```python
from build123d import *

# Parameters (mm, degrees)
F3_D     = 6.5278
F3_DEPTH = 9.525
F3_TIP   = 1.9611489744
F5_D     = 6.5278
F5_DEPTH = 9.525
F5_TIP   = 1.9611489744


with BuildPart() as f1:
    # F0 (on Front) → F1 (revolve)
    with BuildSketch(Plane.XZ):
        with BuildLine():
            Line((-57.0530471623, 106.8800194085), (-82.4530471623, 106.8800194085))
            Line((-82.4530471623, 106.8800194085), (-82.4530471623, -45.5199805915))
            Line((-82.4530471623, -45.5199805915), (-44.3530471623, -45.5199805915))
            Line((-44.3530471623, -45.5199805915), (-44.3530471623, -32.8199805915))
            add(Edge.make_bspline(
                [(-72.9280471623, -20.1199805915), (-72.9280471623, -32.8199805915), (-55.7276420295, -32.8199805915), (-44.3530471623, -32.8199805915)],
                knots=[0, 0, 0, 0, 31.2701235207, 31.2701235207, 31.2701235207, 31.2701235207], degree=3))
            Line((-72.9280471623, -20.1199805915), (-72.9280471623, 81.4800194085))
            ThreePointArc((-72.9280471623, 81.4800194085), (-69.2083032834, 90.4602755295), (-60.2280471623, 94.1800194085))
            Line((-60.2280471623, 94.1800194085), (-57.0530471623, 94.1800194085))
            Line((-57.0530471623, 94.1800194085), (-57.0530471623, 106.8800194085))
        make_face()
    revolve(axis=Axis((-82.4530471623, 0, 30.6800194085), (0, 0, -1)))

    # F3
    with Locations(Plane.XY.offset(106.8800194085)):
        with Locations((-82.4530471623, 15.875), (-82.4530471623, -15.875)):
            Hole(F3_D / 2, depth=F3_DEPTH)
            with Locations((0, 0, -(F3_DEPTH + F3_TIP / 2))):  # 118° drill point
                Cone(0, F3_D / 2, F3_TIP, mode=Mode.SUBTRACT)

    # F5
    with Locations(Plane(origin=(0, 0, -45.5199805915), x_dir=(1, 0, 0), z_dir=(0, 0, -1))):
        with Locations((-82.4530471623, 19.05), (-82.4530471623, -19.05)):
            Hole(F5_D / 2, depth=F5_DEPTH)
            with Locations((0, 0, -(F5_DEPTH + F5_TIP / 2))):  # 118° drill point
                Cone(0, F5_D / 2, F5_TIP, mode=Mode.SUBTRACT)


solid = f1.part
```
Here's how the part is built. I have some questions about the finished solid (model axes, mm). A direction names the side the tool comes from. Round coordinates to 2 decimals unless told otherwise and drop trailing zeros. Loops run counter-clockwise (first coordinate to the right, second up) from the corner with the lowest first, then second, coordinate; pieces in that order, holes last. Notation, with made-up numbers: (76, 18.25) -> (116, 18.25) arc R9 cw to (116, 22.25) -> close; hole circle Ø6 at (7, -4). An arc over 180 degrees is marked (long way). Answer as CSV lines item,"result". Start each with the question number.
1. I'm going to push flat-ended pins straight in: P1, Ø4, axis at x = -82.45, y = -19.05, coming from the +Z side; P2, Ø6, axis at y = -4, z = 68, coming from the -X side; P3, Ø10, axis at x = -101.5, z = 7, coming from the +Y side; P4, Ø5, axis at x = -82.45, y = 15.88, coming from the +Z side. Where does each tip first touch, or does it pass through?
2. Imagine slicing it at A-A on z = 52.5. Write out the boundary of the cut face in (x, y) (3 decimals), plus the area to 3 significant figures.
3. If we mould it in two halves opening along Z, with no side actions, what happens to faces 4 (the face through (-82.3, 22.5, 94.18)), 5 (the face through (-73.368, -2.861, 31.391)), 6 (the face through (-82.576, 19.603, -34.374)), 7 (the face through (-85.566, 16.855, 102.051))? For each: pulls with the +Z half, pulls with the -Z half, needs draft (parallel to the pull), parting line crosses it, or undercut.
4. I need wall thicknesses on probe 1 along Z at (x, y) = (-100, -16.5); probe 2 along X at (y, z) = (19, -43); probe 3 along Z at (x, y) = (-107.5, -22.5). Which ranges of each line are inside material? Lowest first, please. Write a range as from..to.
5. For faces 1 (the face through (-85.566, -20.03, -40.691)), 2 (the face through (-85.566, -14.895, 102.051)), 3 (the face through (-82, -1, -45.52)), which set-ups out of +Z, -Z, +X, -X, +Y, -Y let a thin tool reach every point of the face, with its end or its side?
Solution:
1,P1,"z = 106.88"
1,P2,"x = -91.93"
1,P3,"through"
1,P4,"z = 96.9"
2,outline,"circle Ø19.05 at (-82.453, 0)"
2,area,"285 mm²"
3,face 4,"undercut"
3,face 5,"undercut"
3,face 6,"pulls with the -Z half"
3,face 7,"needs draft"
4,probe 1,"-45.52..-32.15, 94.18..106.88"
4,probe 2,"-115.48..-85.72, -79.19..-49.43"
4,probe 3,"-45.52..-32.8"
5,face 1,"-Z"
5,face 2,"+Z"
5,face 3,"-Z, +X, -X, +Y, -Y"
